Geometry: see drawing. Coordinates: mm, zero at the bounding-box minimum. A direction names the side the tool comes from. Coordinates: 2 decimals unless noted, no trailing zeros. Write each loop counter-clockwise with the first axis right and the second up, starting at its lowest first coordinate (ties: lowest second). Pieces come first, ordered by that corner, then holes. Notation, with made-up numbers: (63, 69.25) - (116, 69.25) arc R21 cw to (116, 78.25) - close; hole circle Ø3 at (85.25, -4). An arc over 180 degrees is marked (long way). One line per question, with ' | ' between items. Start each with the question number.
Q1. Cut plane C-C, the plane x = 12. Return loops of the section in (y, z), plus the area to 3 significant figures.
Q2. Line query: line 1 (Y direction, x = 43, z = 2); line 2 (X direction, y = 32.5, z = 2.55); line 3 (X direction, y = 32, z = 0.65). Output: solid intervals per line, ascending.
Q3. Access query for the marked faces 1 and 2. Directions: +Z, -Z, +X, -X, +Y, -Y. A direction counts if a zero-diameter tool reaches every point of the face in a straight line with its end or side. Return the directions, or none.
Q4. Contact query for flat-ended pins moving along their axis: P1, Ø1.5, axis at y = 28, z = 3.5, coming from the +X side; P2, Ø2.5, axis at x = 56, y = 20, coming from the -Z side; P3, Ø5, axis at x = 16, y = 39, coming from the +Z side. Output: stop coordinate, or through.
Q5. Cut plane A-A, the plane z = 3.15. Return loops of the section in (x, y) (1 decimal).
Q6. Cut plane B-B, the plane y = 29.5. Return loops of the section in (x, z), plus the area to 3 significant figures.
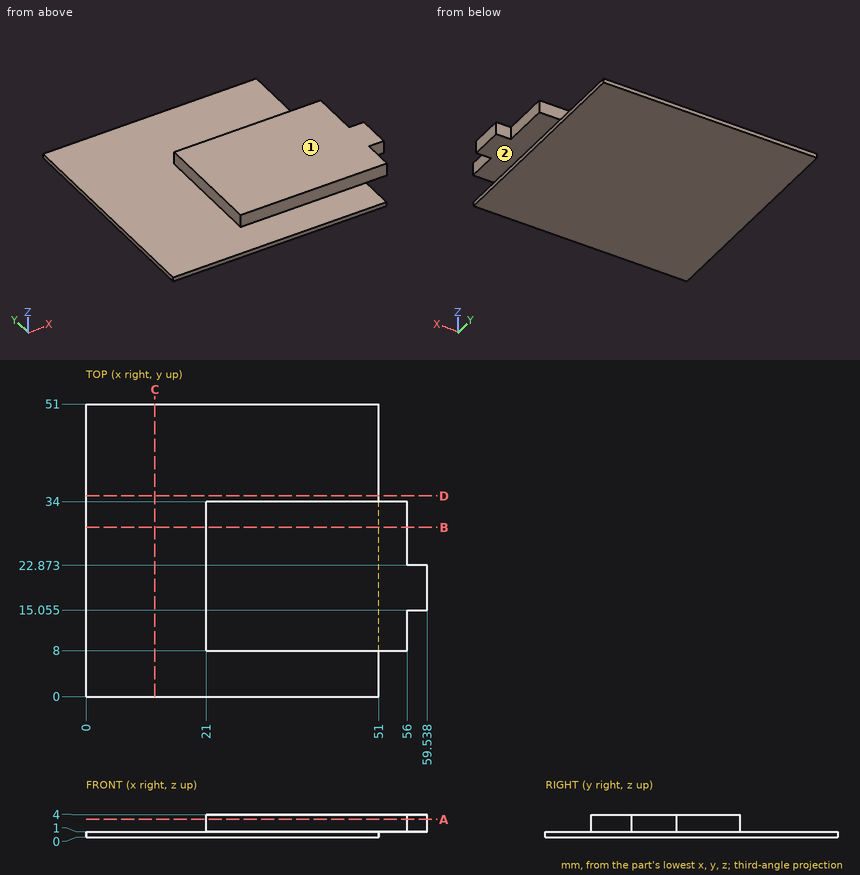
Reply:
1) outline: (0, 0) - (51, 0) - (51, 1) - (0, 1) - close | area: 51.0 mm^2
2) line 1: y = 8 to 34 | line 2: x = 21 to 56 | line 3: x = 0 to 51
3) face 1: +Z, +X, -X, +Y, -Y | face 2: -Z, +X, +Y, -Y
4) P1: stops at x = 56 | P2: stops at z = 1 | P3: stops at z = 1
5) outline: (21, 8) - (56, 8) - (56, 15.1) - (59.5, 15.1) - (59.5, 22.9) - (56, 22.9) - (56, 34) - (21, 34) - close
6) outline: (0, 0) - (51, 0) - (51, 1) - (56, 1) - (56, 4) - (21, 4) - (21, 1) - (0, 1) - close | area: 156 mm^2
